CAD build for the part. Positions are in the model's coordinates, mm. A direction names the side the tool comes from. Round coordinates to 2 decimals unless told otherwise and drop trailing zeros. Write each loop counter-clockwise with the first axis right and the second up, starting at its lowest first coordinate (ties: lowest second). Pieces come first, ordered by that corner, then holes. Notation, with made-up numbers: (-15, 66) - (38, 66) arc R29 cw to (38, 94) - close; hole circle Ø1 at (-34.75, 11). An arc over 180 degrees is marked (long way). Use one line per item in the form item = value. Start each with the question number.
Item 1: Tool access for faces 1 (the flat face through (-0.5, -0.5, 10)), 2 (the flat face through (0, 2, 13.6)), 3 (the flat face through (0, -0.1, 10)): list every direction of +Z, -Z, +X, -X, +Y, -Y with a clear straight run to the whole face (end or side of a thin tool).
Item 2: Band-saw the part on C-C, the plane x = 0. List the corners of the cut face in (y, z), and give its area (3 significant figures).
Item 3: Pin check, flat tips, straight feed: pin 1 (0.8 mm diameter, centred on x = -4, z = 11, fed in from +Y); pin 2 (0.6 mm diameter, centred on y = 2, z = 11, fed in from +X); pin 3 (0.9 mm diameter, centred on y = -0.5, z = 9, fed in from -X). Stop position of each tip, or through.
Item 4: Band-saw the part on D-D, the plane y = 1.7. List the corners of the cut face in (x, z), and give its area (3 significant figures).
Item 5: Drill centre lines: L1, parallel to Y at x = 1.25, z = 12.25; L2, parallel to Y at x = -3, z = 11; L3, parallel to X at y = 5.25, z = 11.75. Where is each one in solid material? Low to high.
Item 6: Pull direction Y, two halves, no side cores. Call faces 4 (the flat face through (-0.028, -0.106, 7.116)), 5 (the cylindrical face through (4.9, 4.2, 11.4)), 6 (the flat face through (2, 7, 9.6)): +Y half, -Y half, draft (parallel to the pull), parting line (faces both ways), or undercut.
Item 7: Band-saw the part on B-B, the plane z = 7.75. List the corners of the cut face in (x, y), and give its area (3 significant figures).
from build123d import *

# Parameters (mm, degrees)
PAD004_DEPTH              = 4
BOX019_W                  = 2
BOX019_H                  = 0.4
BOX019_DEPTH              = 5.7
PAD003_DEPTH              = 4
BOX021_W                  = 2
BOX021_H                  = 0.4
BOX021_DEPTH              = 5.7
BOX020_W                  = 3
BOX020_H                  = 0.4
BOX020_DEPTH              = 4.5
ARRAY_COUNT               = 4
CYLINDER015_R             = 5
CYLINDER015_DEPTH         = 5
CYLINDER019_R             = 6
CYLINDER019_DEPTH         = 1
CYLINDER018_R             = 5.5
CYLINDER018_DEPTH         = 4
FILLET_R                  = 0.3
FUSION001_PLACEMENT_ANGLE = 90


with BuildPart() as pad004:
    # Sketch007 → Pad004 (new body)
    with BuildSketch(Plane(origin=(0.3, -2, 0), x_dir=(-1, 0, 0), z_dir=(0, 1, 0))):
        Polygon((-1.9, 4.62141), (-1.9, -1.87859), (-1.1, -1.07859), (-1.5, -1.07859), (-1.5, 4.62141), align=None)
    extrude(amount=PAD004_DEPTH)


with BuildPart() as cubo008:
    # Box019 → Box019 (new body)
    with BuildSketch(Plane(origin=(-1, -2.2, -1.1), x_dir=(1, 0, 0), z_dir=(0, 0, 1))):
        with Locations((1, 0.2)):
            Rectangle(BOX019_W, BOX019_H)
    extrude(amount=BOX019_DEPTH)


with BuildPart() as pad003:
    # Sketch008 → Pad003 (new body)
    with BuildSketch(Plane.XZ.offset(-2)):
        Polygon((-2.2, 4.62141), (-2.2, -1.87859), (-1.4, -1.07859), (-1.8, -1.07859), (-1.8, 4.62141), align=None)
    extrude(amount=PAD003_DEPTH)


with BuildPart() as cubo007:
    # Box021 → Box021 (new body)
    with BuildSketch(Plane(origin=(-1, 1.8, -1.1), x_dir=(1, 0, 0), z_dir=(0, 0, 1))):
        with Locations((1, 0.2)):
            Rectangle(BOX021_W, BOX021_H)
    extrude(amount=BOX021_DEPTH)


with BuildPart() as array:
    # Box020 → Box020 (new body)
    with BuildSketch(Plane(origin=(2.1, -0.2, 0), x_dir=(1, 0, 0), z_dir=(0, 0, 1))):
        with Locations((1.5, 0.2)):
            Rectangle(BOX020_W, BOX020_H)
    extrude(amount=BOX020_DEPTH)

    # Array: Array ×4 about axis
    array_axis = Axis((0, 0, 0), (0, 0, 1))


with BuildPart() as array_1:
    add(array.part)
    for i in range(1, ARRAY_COUNT):
        add(array.part.rotate(array_axis, i * 360 / ARRAY_COUNT))


with BuildPart() as cilindro018:
    # Cylinder015 → Cylinder015 (new body)
    with BuildSketch(Plane.XY.offset(-0.5)):
        Circle(CYLINDER015_R)
    extrude(amount=CYLINDER015_DEPTH)


with BuildPart() as cilindro017:
    # Cylinder019 → Cylinder019 (new body)
    with BuildSketch(Plane.XY):
        Circle(CYLINDER019_R)
    extrude(amount=CYLINDER019_DEPTH)


with BuildPart() as obj1:
    # Cylinder018 → Cylinder018 (new body)
    with BuildSketch(Plane.XY.offset(1)):
        Circle(CYLINDER018_R)
    extrude(amount=CYLINDER018_DEPTH)

    # Fusion002: union Cilindro017
    add(cilindro017.part)

    # Cut032: cut Cilindro018
    add(cilindro018.part, mode=Mode.SUBTRACT)

    # Fillet
    fillet_edges = [obj1.edges().sort_by_distance(p)[0] for p in [
        (-5.5, 0, 5),
    ]]
    fillet(fillet_edges, radius=FILLET_R)

    # Fusion001: union Pad004, Cubo008, Pad003, Cubo007, Array
    add(pad004.part)
    add(cubo008.part)
    add(pad003.part)
    add(cubo007.part)
    add(array_1.part)


with BuildPart() as obj1_1:
    # Fusion001 placement: moved
    add(obj1.part.moved(Location((0, 1.7, 8.6))).rotate(Axis((0, 1.7, 8.6), (0, 0, 1)), FUSION001_PLACEMENT_ANGLE))


solid = obj1_1.part
Determined:
q1.face_1 = -Z
q1.face_2 = +Z, +X, -X, +Y, -Y
q1.face_3 = none
q2.outline = (-4.3, 8.6) - (-0.5, 8.6) - (-0.5, 6.72) - (0.3, 7.52) - (-0.1, 7.52) - (-0.1, 13.1) - (3.5, 13.1) - (3.5, 7.52) - (3.1, 7.52) - (3.9, 6.72) - (3.9, 8.6) - (7.7, 8.6) - (7.7, 9.6) - (7.2, 9.6) - (7.2, 13.3) arc R0.3 ccw to (6.9, 13.6) - (-3.5, 13.6) arc R0.3 ccw to (-3.8, 13.3) - (-3.8, 9.6) - (-4.3, 9.6) - close
q2.area = 41.3 mm²
q3.pin_1 = 5.86
q3.pin_2 = 5.5
q3.pin_3 = -5.74
q4.outline = (-6, 8.6) - (-2.2, 8.6) - (-2.2, 7.5) - (-1.8, 7.5) - (-1.8, 13.1) - (1.8, 13.1) - (1.8, 7.5) - (2.2, 7.5) - (2.2, 8.6) - (6, 8.6) - (6, 9.6) - (5.5, 9.6) - (5.5, 13.3) arc R0.3 ccw to (5.2, 13.6) - (-5.2, 13.6) arc R0.3 ccw to (-5.5, 13.3) - (-5.5, 9.6) - (-6, 9.6) - close
q4.area = 40.6 mm²
q5.L1 = -3.66 to -3.14, -0.5 to -0.1, 3.5 to 3.9, 6.54 to 7.06
q5.L2 = -2.91 to -2.3, 1.5 to 1.9, 5.7 to 6.31
q5.L3 = -4.2 to -3.52, -0.2 to 0.2, 3.52 to 4.2
q6.face_4 = undercut
q6.face_5 = parting line
q6.face_6 = draft
q7.outline = (-2.2, 0.7) - (-1.8, 0.7) - (-1.8, 2.7) - (-2.2, 2.7) - close; (-2, -0.5) - (2, -0.5) - (2, -0.1) - (-2, -0.1) - close; (-2, 3.5) - (2, 3.5) - (2, 3.9) - (-2, 3.9) - close; (1.8, 0.7) - (2.2, 0.7) - (2.2, 2.7) - (1.8, 2.7) - close
q7.area = 4.80 mm²
